Build history of the part. All positions in model axes, mm. Face numbers are marked on the shaded views. A direction names the side the tool comes from. Round coordinates to 2 decimals unless told otherwise and drop trailing zeros. Write each loop counter-clockwise with the first axis right and the second up, starting at its lowest first coordinate (ties: lowest second). Pieces come first, ordered by that corner, then holes. Notation, with made-up numbers: M -7.75,57 L 0.25,57 A17 cw 0.25,89 Z; hole C 6.25,9 d9. An arc over 180 degrees is marked long. Write item = value, one per line.
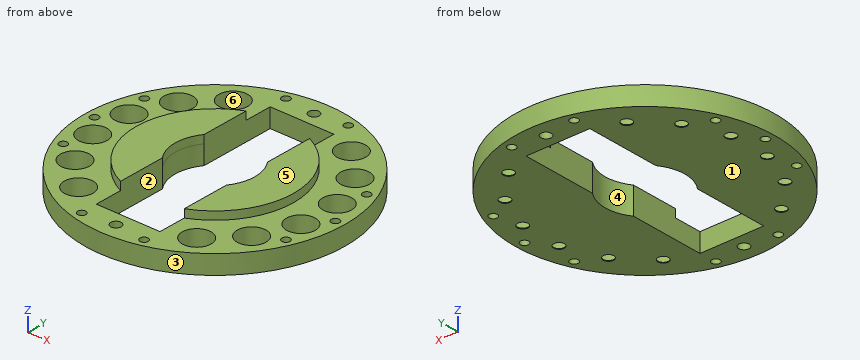
from build123d import *

# Parameters (mm, degrees)
SKETCH1_R                      = 272.79346
SKETCH1_R_2                    = 30.1625
SKETCH1_R_3                    = 8.617585
SKETCH1_R_4                    = 11.00963
SKETCH1_R_5                    = 164.44976
SKETCH1_R_6                    = 83.56346
EXTRUDE5_DEPTH                 = 39.69258
EXTRUDE8_DEPTH                 = 16.97482
SKETCH4_W                      = 134.3533
SKETCH4_H                      = 418.01542
EXTRUDE10_DEPTH                = 64.83223
SKETCH7_R                      = 30.1625
EXTRUDE12_DEPTH                = 1.59258
F_1_8_TAPPED_HOLE1_D           = 22.225
F_1_8_TAPPED_HOLE1_ON_FACE_2_D = 22.225


with BuildPart() as part:
    # Sketch1 → Extrude5 (new body)
    with BuildSketch(Plane.XY):
        Circle(SKETCH1_R)
        with Locations((219.584848865, -43.672962802)):
            Circle(SKETCH1_R_2, mode=Mode.SUBTRACT)
        with Locations((-219.57722315, 43.711286923)):
            Circle(SKETCH1_R_2, mode=Mode.SUBTRACT)
        with Locations((186.220609513, -124.284826602)):
            Circle(SKETCH1_R_2, mode=Mode.SUBTRACT)
        with Locations((-186.220609513, 124.284826602)):
            Circle(SKETCH1_R_2, mode=Mode.SUBTRACT)
        with Locations((124.588226536, -186.017760817)):
            Circle(SKETCH1_R_2, mode=Mode.SUBTRACT)
        with Locations((-124.588226536, 186.017760817)):
            Circle(SKETCH1_R_2, mode=Mode.SUBTRACT)
        with Locations((-124.160317609, -186.303647474)):
            Circle(SKETCH1_R_2, mode=Mode.SUBTRACT)
        with Locations((124.160317609, 186.303647474)):
            Circle(SKETCH1_R_2, mode=Mode.SUBTRACT)
        with Locations((-186.104477248, -124.458656103)):
            Circle(SKETCH1_R_2, mode=Mode.SUBTRACT)
        with Locations((186.104477248, 124.458656103)):
            Circle(SKETCH1_R_2, mode=Mode.SUBTRACT)
        with Locations((219.584848865, 43.672962802)):
            Circle(SKETCH1_R_2, mode=Mode.SUBTRACT)
        with Locations((-219.584848865, -43.672962802)):
            Circle(SKETCH1_R_2, mode=Mode.SUBTRACT)
        with Locations((-234.688092884, -97.272902019)):
            Circle(SKETCH1_R_3, mode=Mode.SUBTRACT)
        with Locations((-65.668151158, -245.414368635)):
            Circle(SKETCH1_R_3, mode=Mode.SUBTRACT)
        with Locations((65.779081624, -245.384658913)):
            Circle(SKETCH1_R_3, mode=Mode.SUBTRACT)
        with Locations((234.735092644, -97.159429242)):
            Circle(SKETCH1_R_3, mode=Mode.SUBTRACT)
        with Locations((-234.564955174, 97.569463528)):
            Circle(SKETCH1_R_3, mode=Mode.SUBTRACT)
        with Locations((-65.668151158, 245.414368635)):
            Circle(SKETCH1_R_3, mode=Mode.SUBTRACT)
        with Locations((65.668151158, 245.414368635)):
            Circle(SKETCH1_R_3, mode=Mode.SUBTRACT)
        with Locations((234.564955174, 97.569463528)):
            Circle(SKETCH1_R_3, mode=Mode.SUBTRACT)
        with Locations((254.04826, 0)):
            Circle(SKETCH1_R_3, mode=Mode.SUBTRACT)
        with Locations((-254.04826, 0)):
            Circle(SKETCH1_R_3, mode=Mode.SUBTRACT)
        with Locations((0, -238.00054)):
            Circle(SKETCH1_R_4, mode=Mode.SUBTRACT)
        with Locations((0, 238.00054)):
            Circle(SKETCH1_R_4, mode=Mode.SUBTRACT)
        Circle(SKETCH1_R_5, mode=Mode.SUBTRACT)
        Circle(SKETCH1_R_5)
        Circle(SKETCH1_R_6, mode=Mode.SUBTRACT)
    extrude(amount=EXTRUDE5_DEPTH)

    # Sketch3 → Extrude8 (add)
    with BuildSketch(Plane.XY.offset(39.69258)):
        with BuildLine():
            Line((-66.9036, 150.950693964), (-66.9036, 50.067555904))
            ThreePointArc((-66.9036, 50.067555904), (-83.56346, 0), (-66.9036, -50.067555904))
            Line((-66.9036, -50.067555904), (-66.9036, -150.950693964))
            ThreePointArc((-66.9036, -150.950693964), (-165.1127, 0), (-66.9036, 150.950693964))
        make_face()
        with BuildLine():
            Line((67.4497, 150.707470522), (67.4497, 49.329401143))
            ThreePointArc((67.4497, 49.329401143), (83.56346, 0), (67.4497, -49.329401143))
            Line((67.4497, -49.329401143), (67.4497, -150.707470522))
            ThreePointArc((67.4497, -150.707470522), (165.1127, 0), (67.4497, 150.707470522))
        make_face()
    extrude(amount=EXTRUDE8_DEPTH)

    # Sketch4 → Extrude10 (cut)
    with BuildSketch(Plane.XY.offset(56.6674)):
        with Locations((0.27305, 0)):
            Rectangle(SKETCH4_W, SKETCH4_H)
    extrude(amount=-EXTRUDE10_DEPTH, mode=Mode.SUBTRACT)

    # Sketch7 → Extrude12 (add)
    with BuildSketch(Plane(origin=(0, 0, 0), x_dir=(-1, 0, 0), z_dir=(0, 0, -1))):
        with Locations((-124.160317609, 186.303647474)):
            Circle(SKETCH7_R)
        with Locations((-186.104477248, 124.458656103)):
            Circle(SKETCH7_R)
        with Locations((-219.584848865, 43.672962802)):
            Circle(SKETCH7_R)
        with Locations((-219.584848865, -43.672962802)):
            Circle(SKETCH7_R)
        with Locations((-186.220609513, -124.284826602)):
            Circle(SKETCH7_R)
        with Locations((-124.588226536, -186.017760817)):
            Circle(SKETCH7_R)
        with Locations((124.160317609, -186.303647474)):
            Circle(SKETCH7_R)
        with Locations((186.104477248, -124.458656103)):
            Circle(SKETCH7_R)
        with Locations((219.584848865, -43.672962802)):
            Circle(SKETCH7_R)
        with Locations((219.57722315, 43.711286923)):
            Circle(SKETCH7_R)
        with Locations((186.220609513, 124.284826602)):
            Circle(SKETCH7_R)
        with Locations((124.588226536, 186.017760817)):
            Circle(SKETCH7_R)
    extrude(amount=-EXTRUDE12_DEPTH)

    # 1-8 Tapped Hole1 (through all)
    with Locations(Plane(origin=(124.160317609, 186.303647474, 39.69258), x_dir=(1, 0, 0), z_dir=(0, 0, 1))):
        with Locations((0, 0), (95.424531256, -142.630684672), (95.424531256, -229.976610276), (62.060291904, -310.588474076), (0.427908927, -372.321408291), (-310.264794857, -310.762303577), (-310.380927122, -62.018820872)):
            Hole(F_1_8_TAPPED_HOLE1_D / 2)

    # 1-8 Tapped Hole1 on face 2 (through all)
    with Locations(Plane(origin=(124.160317609, 186.303647474, 1.59258), x_dir=(1, 0, 0), z_dir=(0, 0, 1))):
        with Locations((0, 0), (61.944159639, -61.844991371), (-248.320635218, -372.607294948), (-343.745166474, -229.976610276), (-343.737540759, -142.592360551), (-248.748544145, -0.285886657)):
            Hole(F_1_8_TAPPED_HOLE1_ON_FACE_2_D / 2)


solid = part.part
1. Mould opens along X. For the marked faces 1, 2 and 3 say: pulls with the +X half, pulls with the -X half, needs draft (parallel to the pull), parting line crosses it, or undercut.
Responses:
face_1 = needs draft
face_2 = undercut
face_3 = parting line crosses it
2. Probe probe 1 along X at (y, z) = (201, 26); probe 2 along X at (y, z) = (-169.5, 5); probe 3 along Z at (x, y) = (187.5, -10.5). List the from-to ranges inside material, lowest first.
Responses:
probe_1 = -184.43 to -150.77, -98.41 to -66.9, 67.45 to 97.82, 150.5 to 184.43
probe_2 = -213.74 to -149.21, -99.11 to -66.9, 67.45 to 99.35, 149.83 to 213.74
probe_3 = 0 to 39.69
3. Tool access for the marked faces 4, 5 and 6: list every direction of +Z, -Z, +X, -X, +Y, -Y with a clear straight run to the whole face (end or side of a thin tool).
Responses:
face_4 = +Z, -Z
face_5 = +Z, +X, -X, +Y, -Y
face_6 = +Z
4. Flat gauge pins, fed straight in: pin 1 (6 mm diameter, centred on y = 175.5, z = 27, fed in from -X); pin 2 (4 mm diameter, centred on x = 207.5, z = 22, fed in from +Y); pin 3 (3 mm diameter, centred on x = 175.5, y = 46, fed in from +Z); pin 4 (18 mm diameter, centred on x = -124.59, y = 186.02, fed in from +Z). Where does each tip first touch, or does it go through?
Responses:
pin_1 = -211.33
pin_2 = 179.4
pin_3 = 39.69
pin_4 = through
5. Band-saw the part on D-D (y = 166). List the corners of the cut face in (x, z).
Responses:
outline = M -216.47,0 L -66.9,0 L -66.9,39.69 L -102.03,39.69 L -102.03,1.59 L -147.15,1.59 L -147.15,39.69 L -216.47,39.69 Z; M 67.45,0 L 216.47,0 L 216.47,39.69 L 146.47,39.69 L 146.47,1.59 L 101.85,1.59 L 101.85,39.69 L 67.45,39.69 Z
6. Band-saw the part on A-A (y = 0). List the corners of the cut face in (x, z).
Responses:
outline = M -272.79,0 L -262.67,0 L -262.67,39.69 L -272.79,39.69 Z; M -245.43,0 L -83.56,0 L -83.56,56.67 L -165.11,56.67 L -165.11,39.69 L -245.43,39.69 Z; M 83.56,0 L 245.43,0 L 245.43,39.69 L 165.11,39.69 L 165.11,56.67 L 83.56,56.67 Z; M 262.67,0 L 272.79,0 L 272.79,39.69 L 262.67,39.69 Z
7. Band-saw the part on B-B (x = 0). List the corners of the cut face in (y, z).
Responses:
outline = M -272.79,0 L -249.01,0 L -249.01,39.69 L -272.79,39.69 Z; M -226.99,0 L -209.01,0 L -209.01,39.69 L -226.99,39.69 Z; M 209.01,0 L 226.99,0 L 226.99,39.69 L 209.01,39.69 Z; M 249.01,0 L 272.79,0 L 272.79,39.69 L 249.01,39.69 Z
8. Band-saw the part on C-C (z = 24). Count the separate pieces of the cut face and the enclosed holes in it, plus the area to 3 significant figures.
Responses:
separate_pieces = 1
enclosed_holes = 25
area = 138,000 mm²
